Part model, mm, in its own coordinate system. Face numbers are marked on the shaded views. A direction names the side the tool comes from. Round coordinates to 2 decimals unless told otherwise and drop trailing zeros. Write each loop counter-clockwise with the first axis right and the second up, starting at its lowest first coordinate (ties: lowest second). Pieces come first, ordered by that corner, then holes. Notation, with made-up numbers: M 32.25,-15 L 43.25,-15 A21 cw 43.25,12 Z; hole C 33,4 d3. An arc over 180 degrees is marked long. Use a Markdown table: item, result. Add a question column.
1) Which spindle directions (+Z, -Z, +X, -X, +Y, -Y) get a long thin tool onto all of the face, cutting with end or side? Do the marked faces 1 and 2. Say none if no direction does.
2) Slice it at C-C on x = -34. Write the cut outline in (y, z), plus the area to 3 significant figures.
3) Wall check: probe 1 along Y at (x, z) = (0.7, 22.7); probe 2 along Z at (x, y) = (-39.5, -5.5); probe 3 along X at (y, z) = (-13, 2). Give the ranges that are in metal, low to high.
4) Slice it at A-A on y = 15. Write the cut outline in (x, z).
5) Drop flat-ended pins along their axis: P1, Ø6.5, axis at y = 15, z = 27.7, coming from the -X side; P2, Ø16, axis at x = -30.5, y = -5.5, coming from the +Z side. Give the stop position or say it passes through.
6) Slice it at D-D on y = 24. Write the cut outline in (x, z), plus the area to 3 significant figures.
7) Slice it at B-B on z = 27.7. Write the cut outline in (x, y).
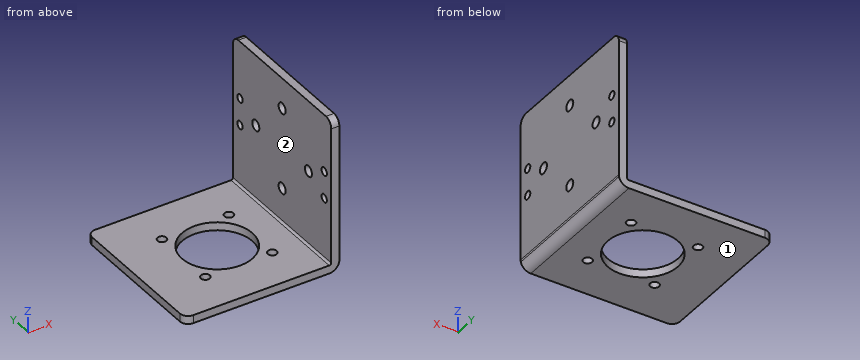
```python
from build123d import *

# Parameters (mm, degrees)
SKETCH_2_W             = 110
SKETCH_2_H             = 56
SM_BASE_FLANGE_1_DEPTH = 3
OTHER_START            = -28
OTHER_1_DEPTH          = 56
OTHER_1_2_DEPTH        = 56
SKETCH_8_R             = 2
CUT_EXTRUDE_1_DEPTH    = 10
FILLET_1_R             = 3
SKETCH_9_R             = 13
CUT_EXTRUDE_2_DEPTH    = 10
SKETCH_10_R            = 1.65
CUT_EXTRUDE_3_DEPTH    = 82.992914788
SKETCH_11_R            = 1.5
CUT_EXTRUDE_4_DEPTH    = 10


# Read off the part's stored shape, not the designer's step: 绘制的折弯1
# Sheet-metal steps are written as plain solids
with BuildPart() as part:
    # Sketch 2 → 基体-法兰1 (new body)
    with BuildSketch(Plane.XY):
        Rectangle(SKETCH_2_W, SKETCH_2_H)
    extrude(amount=-SM_BASE_FLANGE_1_DEPTH)

    # Other 1 outline → Other 1 (cut)
    with BuildSketch(Plane(origin=(0, 0, 0), x_dir=(1, 0, 0), z_dir=(0, 1, 0)).offset(OTHER_START)):
        with BuildLine():
            ThreePointArc((-1.756621532, 3), (0.610845469, 2.154295979), (1.906655689, 0))
            Line((1.906655689, 0), (55, 0))
            Line((55, 0), (55, 3))
            Line((55, 3), (-1.756621532, 3))
        make_face()
    extrude(amount=OTHER_1_DEPTH, mode=Mode.SUBTRACT)

    # Other 1 2 outline → Other 1 2 (add)
    with BuildSketch(Plane(origin=(0, 0, 0), x_dir=(1, 0, 0), z_dir=(0, 1, 0)).offset(OTHER_START)):
        with BuildLine():
            Line((-1.020021532, -0.7366), (-1.020021532, -53.979978468))
            Line((-1.020021532, -53.979978468), (1.979978468, -53.979978468))
            Line((1.979978468, -53.979978468), (1.979978468, -0.7366))
            ThreePointArc((1.979978468, -0.7366), (1.961602589, -0.36647982), (1.906655689, 0))
            Line((1.906655689, 0), (-1.756621532, 0))
            ThreePointArc((-1.756621532, 0), (-1.235766677, -0.215745145), (-1.020021532, -0.7366))
        make_face()
    extrude(amount=OTHER_1_2_DEPTH)

    # 草图8 → 切除-拉伸1 (cut)
    with BuildSketch(Plane.ZY.offset(1.020021532)):
        with Locations((12.7, 0)):
            Circle(SKETCH_8_R)
        with Locations((42.7, 0)):
            Circle(SKETCH_8_R)
        with Locations((27.7, 15)):
            Circle(SKETCH_8_R)
        with Locations((27.7, -15)):
            Circle(SKETCH_8_R)
    extrude(amount=-CUT_EXTRUDE_1_DEPTH, mode=Mode.SUBTRACT)

    # 圆角1
    fillet_1_edges = [part.edges().sort_by_distance(p)[0] for p in [
        (-55, -28, -1.5),
        (-55, 28, -1.5),
        (0.479978468, -28, 53.979978468),
        (0.479978468, 28, 53.979978468),
    ]]
    fillet(fillet_1_edges, radius=FILLET_1_R)

    # 草图9 → 切除-拉伸2 (cut)
    with BuildSketch(Plane.XY):
        with Locations((-25.020021532, 0)):
            Circle(SKETCH_9_R)
    extrude(amount=-CUT_EXTRUDE_2_DEPTH, mode=Mode.SUBTRACT)

    # 草图10 → 切除-拉伸3 (cut, through all)
    with BuildSketch(Plane.XY):
        with Locations((-12.645652861, 12.374368671)):
            Circle(SKETCH_10_R)
        with Locations((-12.645652861, -12.374368671)):
            Circle(SKETCH_10_R)
        with Locations((-37.394390203, -12.374368671)):
            Circle(SKETCH_10_R)
        with Locations((-37.394390203, 12.374368671)):
            Circle(SKETCH_10_R)
    extrude(amount=-CUT_EXTRUDE_3_DEPTH, mode=Mode.SUBTRACT)

    # 草图11 → 切除-拉伸4 (cut)
    with BuildSketch(Plane(origin=(1.979978468, 0, 0), x_dir=(0, 0, -1), z_dir=(1, 0, 0))):
        with Locations((-32.7, 24)):
            Circle(SKETCH_11_R)
        with Locations((-22.7, 24)):
            Circle(SKETCH_11_R)
    cut_extrude_4 = extrude(amount=-CUT_EXTRUDE_4_DEPTH, mode=Mode.SUBTRACT)

    # 镜向1: 切除-拉伸4 across plane
    add(cut_extrude_4.mirror(Plane.ZX), mode=Mode.SUBTRACT)


solid = part.part
```
Entries:
| question | item | result |
|---|---|---|
| 1 | face 1 | -Z, +X, -X, +Y, -Y |
| 1 | face 2 | +Z, -X, +Y, -Y |
| 2 | outline | M -28,-3 L -9.4,-3 L -9.4,0 L -28,0 Z; M 9.4,-3 L 28,-3 L 28,0 L 9.4,0 Z |
| 2 | area | 112 mm^2 |
| 3 | probe 1 | y = -28 to -25.5, -22.5 to 22.5, 25.5 to 28 |
| 3 | probe 2 | z = -3 to 0 |
| 3 | probe 3 | x = -1.02 to 1.98 |
| 4 | outline | M -55,-3 L -1.76,-3 A3.74 ccw 1.98,0.74 L 1.98,25.7 L -1.02,25.7 L -1.02,0.74 A0.74 cw -1.76,0 L -55,0 Z; M -1.02,29.7 L 1.98,29.7 L 1.98,53.98 L -1.02,53.98 Z |
| 5 | P1 | stops at x = -1.02 |
| 5 | P2 | stops at z = 0 |
| 6 | outline | M -55,-3 L -1.76,-3 A3.74 ccw 1.98,0.74 L 1.98,21.2 L -1.02,21.2 L -1.02,0.74 A0.74 cw -1.76,0 L -55,0 Z; M -1.02,24.2 L 1.98,24.2 L 1.98,31.2 L -1.02,31.2 Z; M -1.02,34.2 L 1.98,34.2 L 1.98,53.98 L -1.02,53.98 Z |
| 6 | area | 312 mm^2 |
| 7 | outline | M -1.02,-28 L 1.98,-28 L 1.98,-17 L -1.02,-17 Z; M -1.02,-13 L 1.98,-13 L 1.98,13 L -1.02,13 Z; M -1.02,17 L 1.98,17 L 1.98,28 L -1.02,28 Z |
